from build123d import *

# Parameters (mm, degrees)
ESBO_O1_W                = 400
ESBO_O1_H                = 400
ESBO_O1_R                = 30
RESSALTO_EXTRUS_O1_DEPTH = 30
RESSALTO_EXTRUS_O2_START = 130
ESBO_O2_R                = 15
RESSALTO_EXTRUS_O2_DEPTH = 30
ESBO_O3_R                = 8
CORTE_EXTRUS_O1_DEPTH    = 93.5


with BuildPart() as part:
    # Esboço1 → Ressalto-extrusão1 (new body)
    with BuildSketch(Plane(origin=(0, 0, 0), x_dir=(1, 0, 0), z_dir=(0, 1, 0))):
        Rectangle(ESBO_O1_W, ESBO_O1_H)
        Circle(ESBO_O1_R, mode=Mode.SUBTRACT)
    extrude(amount=RESSALTO_EXTRUS_O1_DEPTH)

    # Esboço2 → Ressalto-extrusão2 (add)
    with BuildSketch(Plane(origin=(0, 0, 0), x_dir=(0, 0, -1), z_dir=(1, 0, 0)).offset(RESSALTO_EXTRUS_O2_START)):
        with BuildLine():
            Line((-19.485571585, -51.25), (-44.744645862, -7.5))
            ThreePointArc((-44.744645862, -7.5), (-50.235026919, -2.009618943), (-57.735026919, 0))
            Line((-57.735026919, 0), (57.735026919, 0))
            ThreePointArc((57.735026919, 0), (50.235026919, -2.009618943), (44.744645862, -7.5))
            Line((44.744645862, -7.5), (19.485571585, -51.25))
            ThreePointArc((19.485571585, -51.25), (0, -62.5), (-19.485571585, -51.25))
        make_face()
        with Locations((0, -40)):
            Circle(ESBO_O2_R, mode=Mode.SUBTRACT)
    ressalto_extrus_o2 = extrude(amount=RESSALTO_EXTRUS_O2_DEPTH)

    # Espelhar1: Ressalto-extrusão2 across plane
    add(ressalto_extrus_o2.mirror(Plane(origin=(0, 0, 0), x_dir=(0, 0, 1), z_dir=(1, 0, 0))))

    # Esboço3 → Corte-extrusão1 (cut, through all)
    with BuildSketch(Plane(origin=(0, 30, 0), x_dir=(1, 0, 0), z_dir=(0, 1, 0))):
        with Locations((-86.974, 86.974)):
            Circle(ESBO_O3_R)
        with Locations((86.974, 86.974)):
            Circle(ESBO_O3_R)
        with Locations((86.974, -86.974)):
            Circle(ESBO_O3_R)
        with Locations((-86.974, -86.974)):
            Circle(ESBO_O3_R)
    extrude(amount=-CORTE_EXTRUS_O1_DEPTH, mode=Mode.SUBTRACT)


solid = part.part
Work out the finished part from the listing and answer in its coordinate system (mm). A direction names the side the tool comes from. Coordinates: 2 decimals unless noted, no trailing zeros. Write each loop counter-clockwise with the first axis right and the second up, starting at its lowest first coordinate (ties: lowest second). Pieces come first, ordered by that corner, then holes.
1. The part is cut by section B-B, the plane z = 0. Write down the section's boundary in (x, y).
Results list:
outline: (-200, 0) - (-160, 0) - (-160, -25) - (-130, -25) - (-130, 0) - (-30, 0) - (-30, 30) - (-200, 30) - close; (-160, -62.5) - (-130, -62.5) - (-130, -55) - (-160, -55) - close; (30, 0) - (130, 0) - (130, -25) - (160, -25) - (160, 0) - (200, 0) - (200, 30) - (30, 30) - close; (130, -62.5) - (160, -62.5) - (160, -55) - (130, -55) - close
2. Flat-ended cylindrical pins translate along their axes: pin 1 (21 mm diameter, centred on x = -86.974, z = -86.974, fed in from +Y); pin 2 (1.5 mm diameter, centred on x = 9.5, z = -134, fed in from -Y); pin 3 (19 mm diameter, centred on y = -36.5, z = 26.5, fed in from -X); pin 4 (13 mm diameter, centred on x = 86.974, z = 86.974, fed in from +Y). Find the tip coordinate at first contact, or state that the pin passes through.
Results list:
pin 1: stops at y = 30
pin 2: stops at y = 0
pin 3: stops at x = -160
pin 4: passes through
3. For a pull along Z with two mould halves and no side action, classify faces 3 (the cylindrical face through (144.8, -62.5, -0.3)), 4 (the flat face through (144.79, -29.07, -32.29)), 5 (the cylindrical face through (-144.79, -25.128, 1.953)) as +Z half, -Z half, draft (parallel to the pull), parting line (faces both ways), or undercut.
Results list:
face 3: parting line
face 4: -Z half
face 5: undercut
4. For faces 1 (the cylindrical face through (94.364, 15.21, -83.91)), 2 (the flat face through (-130, -24, -1)), determine the directions among +Z, -Z, +X, -X, +Y, -Y from which every point of the face is accessible in a straight line to the end or side of a thin tool.
Results list:
face 1: +Y, -Y
face 2: +Z, -Z, -Y
5. The part is cut by section D-D, the plane y = -40. Write down the section's boundary in (x, z).
Results list:
outline: (-160, -25.98) - (-130, -25.98) - (-130, -15) - (-160, -15) - close; (-160, 15) - (-130, 15) - (-130, 25.98) - (-160, 25.98) - close; (130, -25.98) - (160, -25.98) - (160, -15) - (130, -15) - close; (130, 15) - (160, 15) - (160, 25.98) - (130, 25.98) - close
6. The part is cut by section C-C, the plane y = -13. Write down the section's boundary in (x, z), and give its area (3 significant figures).
Results list:
outline: (-160, -41.57) - (-130, -41.57) - (-130, 41.57) - (-160, 41.57) - close; (130, -41.57) - (160, -41.57) - (160, 41.57) - (130, 41.57) - close
area: 4,990 mm2
7. The part is cut by section A-A, the plane x = 0. Write down the section's boundary in (y, z).
Results list:
outline: (0, -200) - (30, -200) - (30, -30) - (0, -30) - close; (0, 30) - (30, 30) - (30, 200) - (0, 200) - close
8. Consider line 1 along Z through (x, y) = (0, 7.75); line 2 along Y through (x, z) = (-138.75, 0). Determine where each line is inside the solid, lowest interval first.
Results list:
line 1: z = -200 to -30, 30 to 200
line 2: y = -62.5 to -55, -25 to 30
